from build123d import *

# Parameters (mm, degrees)
SKETCH_1_R             = 13
EXTRUDE_1_DEPTH        = 14
EXTRUDE_2_DEPTH        = 71
SKETCH_5_R             = 13
CUT_EXTRUDE_3_DEPTH    = 420.252591423
PATTERN_LINEAR_1_COUNT = 4
PATTERN_LINEAR_1_PITCH = 80
SKETCH_7_W             = 85
SKETCH_7_H             = 320
EXTRUDE_3_DEPTH        = 14
EXTRUDE_4_DEPTH        = 14


with BuildPart() as part:
    # 草图1 → 凸台-拉伸1 (new body)
    with BuildSketch(Plane.XY):
        Polygon((-119.656440364, -63.376666372), (-119.656440364, 256.623333628), (40.343559636, 346.623333628), (100.343559636, 286.623333628), (100.343559636, 71.623333628), align=None)
        with Locations((-16.318215015, 232.316337145)):
            Circle(SKETCH_1_R, mode=Mode.SUBTRACT)
        with Locations((36.830892091, 292.109082639)):
            Circle(SKETCH_1_R, mode=Mode.SUBTRACT)
    extrude(amount=EXTRUDE_1_DEPTH)

    # 草图3 → 凸台-拉伸2 (add)
    with BuildSketch(Plane.XY.offset(14)):
        Polygon((-105.656440364, 264.498333628), (-105.656440364, -54.785757281), (-119.656440364, -63.376666372), (-119.656440364, 256.623333628), align=None)
    extrude(amount=EXTRUDE_2_DEPTH)

    # 草图5 → 切除-拉伸3 (cut, through all)
    with BuildSketch(Plane.ZY.offset(119.656440364)):
        with Locations(Location((47, 216.623333628, 0), (0, 0, 270))):
            Circle(SKETCH_5_R)
    cut_extrude_3 = extrude(amount=-CUT_EXTRUDE_3_DEPTH, mode=Mode.SUBTRACT)

    # 阵列(线性)1: 切除-拉伸3 ×4
    with Locations(*[(0, -i * PATTERN_LINEAR_1_PITCH, 0) for i in range(1, PATTERN_LINEAR_1_COUNT)]):
        add(cut_extrude_3, mode=Mode.SUBTRACT)

    # 草图7 → 凸台-拉伸3 (add)
    with BuildSketch(Plane.ZY.offset(119.656440364)):
        with Locations((42.5, 96.623333628)):
            Rectangle(SKETCH_7_W, SKETCH_7_H)
    extrude(amount=-EXTRUDE_3_DEPTH)

    # 草图8 → 凸台-拉伸4 (add)
    with BuildSketch(Plane.XY.offset(14)):
        Polygon((-119.656440364, 256.623333628), (40.343559636, 346.623333628), (100.343559636, 286.623333628), (100.343559636, 71.623333628), (-119.656440364, -63.376666372), align=None)
    extrude(amount=-EXTRUDE_4_DEPTH)


solid = part.part
CAD build for the part. Positions are in the model's coordinates, mm. A direction names the side the tool comes from. Round coordinates to 2 decimals unless told otherwise and drop trailing zeros. Write each loop counter-clockwise with the first axis right and the second up, starting at its lowest first coordinate (ties: lowest second). Pieces come first, ordered by that corner, then holes. Notation, with made-up numbers: (-33.5, 13.5) -> (-0.5, 13.5) arc R26 ccw to (-0.5, 40.5) -> close; hole circle Ø1 at (4, 37.5). An arc over 180 degrees is marked (long way). Answer as a JSON object with one key per item and string values.
(1) Band-saw the part on D-D, the plane y = 64. List the corners of the cut face in (x, z), then the cut area to 3 significant figures.
Reported:
{"outline": "(-119.66, 0) -> (87.92, 0) -> (87.92, 14) -> (-105.66, 14) -> (-105.66, 85) -> (-119.66, 85) -> close", "area": "3,900 mm^2"}
(2) Band-saw the part on A-A, the plane y = 156. List the corners of the cut face in (x, z).
Reported:
{"outline": "(-119.66, 0) -> (100.34, 0) -> (100.34, 14) -> (-105.66, 14) -> (-105.66, 85) -> (-119.66, 85) -> close"}
(3) Pin check, flat tips, straight feed: P1, Ø2, axis at x = 36, y = 197, coming from the +Z side; P2, Ø4, axis at y = -2.5, z = 62.5, coming from the +X side. Stop position of each tip, or through.
Reported:
{"P1": "stops at z = 14", "P2": "stops at x = -105.66"}
(4) Band-saw the part on B-B, the plane z = 29.5. List the corners of the cut face in (x, y).
Reported:
{"outline": "(-119.66, -63.38) -> (-105.66, -63.38) -> (-105.66, 264.5) -> (-119.66, 256.62) -> close"}
(5) Which spindle directions (+Z, -Z, +X, -X, +Y, -Y) get a long thin tool onto all of the face, cutting with end or side? Do faces 1 (the face through (-1, 149, 14)), 2 (the face through (-11, 139, 0)). Say none if no direction does.
Reported:
{"face 1": "+Z, +X, +Y, -Y", "face 2": "-Z, +X, -X, +Y, -Y"}
(6) Probe probe 1 along Z at (x, y) = (-19.5, 308.5); probe 2 along X at (y, z) = (219, 32.5); probe 3 along Y at (x, z) = (46, 5). List the from-to ranges inside material, lowest first. Write a range as [from, to].
Reported:
{"probe 1": "z = [0, 14]", "probe 2": "x = [-119.66, -105.66]", "probe 3": "y = [38.28, 340.97]"}
(7) Band-saw the part on C-C, the plane x = -91.5. List the corners of the cut face in (y, z), then the cut area to 3 significant figures.
Reported:
{"outline": "(-46.1, 0) -> (272.46, 0) -> (272.46, 14) -> (-46.1, 14) -> close", "area": "4,460 mm^2"}
